```python
from build123d import *

# Parameters (mm, degrees)
SZKIC1_R                        = 20
SZKIC1_R_2                      = 4
DODANIE_WYCI_GNI_CIE1_DEPTH     = 50
WYTNIJ_WYCI_GNI_CIE1_START      = -14.5
WYTNIJ_WYCI_GNI_CIE1_DEPTH      = 14.5
WYTNIJ_WYCI_GNI_CIE2_DEPTH      = 59.479398082
WYTNIJ_WYCI_GNI_CIE2_DEPTH_BACK = 59.479398082
SZKIC3_R                        = 1.75
SZKIC4_W                        = 16
SZKIC4_H                        = 8
WYTNIJ_WYCI_GNI_CIE3_DEPTH      = 68.082039489
SZKIC6_W                        = 20
SZKIC6_H                        = 6
SFAZOWANIE1_SIZE                = 2
WYTNIJ_WYCI_GNI_CIE4_DEPTH      = 58.445626622
WYTNIJ_WYCI_GNI_CIE4_DEPTH_BACK = 58.445626622
SZKIC7_R                        = 2.5
SFAZOWANIE2_SIZE                = 1


with BuildPart() as part:
    # Szkic1 → Dodanie-wyciągnięcie1 (new body)
    with BuildSketch(Plane.XY):
        Circle(SZKIC1_R)
        Circle(SZKIC1_R_2, mode=Mode.SUBTRACT)
    extrude(amount=DODANIE_WYCI_GNI_CIE1_DEPTH)

    # Szkic2 → Wytnij-wyciągnięcie1 (cut)
    with BuildSketch(Plane.XY.offset(50).offset(WYTNIJ_WYCI_GNI_CIE1_START)):
        with BuildLine():
            Line((4.664761516, 2.8), (10.2, 2.8))
            Line((10.2, 2.8), (10.2, 6.2))
            Line((10.2, 6.2), (-10.2, 6.2))
            Line((-10.2, 6.2), (-10.2, 2.8))
            Line((-10.2, 2.8), (-4.664761516, 2.8))
            ThreePointArc((-4.664761516, 2.8), (-3.840140391, 2.365685425), (-3.731809213, 1.44))
            ThreePointArc((-3.731809213, 1.44), (0, -4), (3.731809213, 1.44))
            ThreePointArc((3.731809213, 1.44), (3.840140391, 2.365685425), (4.664761516, 2.8))
        make_face()
    extrude(amount=WYTNIJ_WYCI_GNI_CIE1_DEPTH, mode=Mode.SUBTRACT)

    # Szkic3 → Wytnij-wyciągnięcie2 (cut, two sides: drawn at the far end of the back side and taken through both)
    with BuildSketch(Plane(origin=(0, 2.8, 0), x_dir=(1, 0, 0), z_dir=(0, 1, 0)).offset(-WYTNIJ_WYCI_GNI_CIE2_DEPTH_BACK)):
        with Locations(Location((-8, -46.5, 0), (0, 0, 180))):
            Circle(SZKIC3_R)
        with Locations(Location((-8, -39.5, 0), (0, 0, 180))):
            Circle(SZKIC3_R)
        with Locations(Location((8, -46.5, 0), (0, 0, 180))):
            Circle(SZKIC3_R)
        with Locations(Location((8, -39.5, 0), (0, 0, 180))):
            Circle(SZKIC3_R)
    extrude(amount=WYTNIJ_WYCI_GNI_CIE2_DEPTH + WYTNIJ_WYCI_GNI_CIE2_DEPTH_BACK, mode=Mode.SUBTRACT)

    # Szkic4 → Wytnij-wyciągnięcie3 (cut, through all)
    with BuildSketch(Plane(origin=(20, 0, 0), x_dir=(0, 0, -1), z_dir=(1, 0, 0))):
        with Locations((-42, -16)):
            Rectangle(SZKIC4_W, SZKIC4_H)
    extrude(amount=-WYTNIJ_WYCI_GNI_CIE3_DEPTH, mode=Mode.SUBTRACT)

    # Szkic6 → Wycięcie-obrót1 (revolve, cut)
    with BuildSketch(Plane(origin=(0, 0, 0), x_dir=(0, 0, -1), z_dir=(1, 0, 0)), mode=Mode.PRIVATE) as wyci_cie_obr_t1_sk:
        with Locations((-15, 17)):
            Rectangle(SZKIC6_W, SZKIC6_H)
    revolve(wyci_cie_obr_t1_sk.sketch.rotate(Axis((0, 0, 0), (0, 0, 1)), 90), axis=Axis((0, 0, 0), (0, 0, 1)), mode=Mode.SUBTRACT)

    # Sfazowanie1
    sfazowanie1_edges = [part.edges().sort_by_distance(p)[0] for p in [
        (14, 0, 25),
        (14, 0, 5),
    ]]
    chamfer(sfazowanie1_edges, length=SFAZOWANIE1_SIZE)

    # Szkic7 → Wytnij-wyciągnięcie4 (cut, two sides: drawn at the far end of the back side and taken through both)
    with BuildSketch(Plane(origin=(0, 0, 0), x_dir=(0, 0, -1), z_dir=(1, 0, 0)).offset(-WYTNIJ_WYCI_GNI_CIE4_DEPTH_BACK)):
        with Locations((-15, 0)):
            Circle(SZKIC7_R)
    extrude(amount=WYTNIJ_WYCI_GNI_CIE4_DEPTH + WYTNIJ_WYCI_GNI_CIE4_DEPTH_BACK, mode=Mode.SUBTRACT)

    # Sfazowanie2
    sfazowanie2_edges = [part.edges().sort_by_distance(p)[0] for p in [
        (0, -12, 34),
    ]]
    chamfer(sfazowanie2_edges, length=SFAZOWANIE2_SIZE)


solid = part.part
```
Work out the finished part from the listing and answer in its coordinate system (mm). A direction names the side the tool comes from. Give positions to 0.01 mm unless a question says otherwise; leave off trailing zeros. Order: outer loops, then holes, each group sorted by start corner. A loop starts at its lowest first (then second) coordinate and runs counter-clockwise, first axis right, second up. Notation, with made-up numbers: M 73.25,46.5 L 97.25,46.5 A25 cw 97.25,70.5 Z; hole C 78.25,65.5 d2. An arc over 180 degrees is marked long. Return JSON: item names as keys, results as strings.
1) Section C-C, the plane z = 46.5 is taken. Write down the section's boundary in (x, y), plus the area to 3 significant figures.
Resolved:
{"outline": "M -16,-12 L -9.75,-12 L -9.75,2.8 L -10.2,2.8 L -10.2,6.2 L -9.75,6.2 L -9.75,17.46 A20 ccw Z; M -6.25,-12 L 6.25,-12 L 6.25,2.8 L 4.66,2.8 A1 ccw 3.73,1.44 A4 cw long -3.73,1.44 A1 ccw -4.66,2.8 L -6.25,2.8 Z; M -6.25,6.2 L 6.25,6.2 L 6.25,19 A20 ccw -6.25,19 Z; M 9.75,-12 L 16,-12 A20 ccw 9.75,17.46 L 9.75,6.2 L 10.2,6.2 L 10.2,2.8 L 9.75,2.8 Z", "area": "773 mm^2"}
2) A tool of negligible diameter and unlimited length cuts with its end or side. For faces 4 (the flat face through (-8.98, -13.43, 25)), 5 (the flat face through (0, -16, 34)), 6 (the cylindrical face through (-3.85, 2.38, 42.65)), 7 (the cylindrical face through (8.38, -4.7, 37.79)), 8 (the cylindrical face through (-0.867, -3.905, 24.65)), from which of +Z, -Z, +X, -X, +Y, -Y can it reach the whole face along a straight path? Write none if from no direction.
Resolved:
{"face 4": "none", "face 5": "+Z, +X, -X, -Y", "face 6": "+Z", "face 7": "+Y, -Y", "face 8": "+Z, -Z"}
3) Section A-A, the plane x = 0 is taken. Write down the section's boundary in (y, z), plus the area to 3 significant figures.
Resolved:
{"outline": "M -20,0 L -4,0 L -4,50 L -12,50 L -12,35 L -13,34 L -20,34 L -20,25 L -16,25 L -14,23 L -14,7 L -16,5 L -20,5 Z; M 4,0 L 20,0 L 20,5 L 16,5 L 14,7 L 14,23 L 16,25 L 20,25 L 20,50 L 6.2,50 L 6.2,35.5 L 4,35.5 Z", "area": "1,210 mm^2"}
4) Section B-B, the plane y = 0 is taken. Give the number of separate pieces and of enclosed holes in the cut face, plus the area to 3 significant figures.
Resolved:
{"separate pieces": "4", "enclosed holes": "4", "area": "1,230 mm^2"}
5) Section D-D, the plane z = 15 is taken. Write down the section's boundary in (x, y).
Resolved:
{"outline": "M -13.77,-2.5 A14 ccw 13.77,-2.5 L 3.12,-2.5 A4 cw -3.12,-2.5 Z; M -13.77,2.5 L -3.12,2.5 A4 cw 3.12,2.5 L 13.77,2.5 A14 ccw Z"}
6) For a pull along X with two mould halves and no side action, classify faces 1 (the cylindrical face through (-6.25, 12.51, 46.58)), 2 (the cylindrical face through (-2.6, 19.83, 37.33)), 3 (the flat face through (0, -12, 43)) as +X half, -X half, draft (parallel to the pull), parting line (faces both ways), or undercut.
Resolved:
{"face 1": "undercut", "face 2": "parting line", "face 3": "draft"}
7) Each of these flat-tipped pins is pushed along its axis until it touches: pin 1 (6 mm diameter, centred on x = -6.5, z = 39.5, fed in from +Y); pin 2 (2.5 mm diameter, centred on y = 3.5, z = 43, fed in from -X); pin 3 (1.5 mm diameter, centred on x = -2.5, z = 27, fed in from -Y). Where does it stop, or does it pass through?
Resolved:
{"pin 1": "y = 19.69", "pin 2": "x = -19.87", "pin 3": "y = -19.92"}
8) Straight lines are drawn through the part: line 1 along Z through (x, y) = (8, 10.5); line 2 along Z through (x, y) = (2.5, -18); line 3 along Z through (x, y) = (8, 0). For each, find the intervals that lie inside material, in ascending order. Write a range as [from, to].
Resolved:
{"line 1": "[0, 37.75], [41.25, 44.75], [48.25, 50]", "line 2": "[0, 5], [25, 34]", "line 3": "[0, 12.5], [17.5, 37.75], [41.25, 44.75], [48.25, 50]"}
